from build123d import *

# Parameters (mm, degrees)
F1_DEPTH = 944.626
F2_W     = 12.7
F2_H     = 838.2
F3_DEPTH = 349.25
F4_W     = 368.3
F4_H     = 184.15
F4_R     = 20.6375
F4_W_2   = 247.65
F5_DEPTH = 25.4


with BuildPart() as f1:
    # F0 (on Right) → F1 (new body, symmetric)
    with BuildSketch(Plane.YZ):
        with BuildLine():
            Line((400.05, 361.95), (0, 361.95))
            Line((0, 361.95), (-400.05, 361.95))
            ThreePointArc((-400.05, 361.95), (-422.50064, 352.65064), (-431.8, 330.2))
            Line((-431.8, 330.2), (-431.8, 31.75))
            ThreePointArc((-431.8, 31.75), (-437.379616, 18.279616), (-450.85, 12.7))
            Line((-450.85, 12.7), (-558.8, 12.7))
            Line((-558.8, 12.7), (-558.8, 6.35))
            Line((-558.8, 6.35), (-558.8, 0))
            Line((-558.8, 0), (-450.85, 0))
            ThreePointArc((-450.85, 0), (-428.39936, 9.29936), (-419.1, 31.75))
            Line((-419.1, 31.75), (-419.1, 330.2))
            ThreePointArc((-419.1, 330.2), (-413.520384, 343.670384), (-400.05, 349.25))
            Line((-400.05, 349.25), (0, 349.25))
            Line((0, 349.25), (400.05, 349.25))
            ThreePointArc((400.05, 349.25), (413.520384, 343.670384), (419.1, 330.2))
            Line((419.1, 330.2), (419.1, 31.75))
            ThreePointArc((419.1, 31.75), (428.39936, 9.29936), (450.85, 0))
            Line((450.85, 0), (558.8, 0))
            Line((558.8, 0), (558.8, 6.35))
            Line((558.8, 6.35), (558.8, 12.7))
            Line((558.8, 12.7), (450.85, 12.7))
            ThreePointArc((450.85, 12.7), (437.379616, 18.279616), (431.8, 31.75))
            Line((431.8, 31.75), (431.8, 330.2))
            ThreePointArc((431.8, 330.2), (422.50064, 352.65064), (400.05, 361.95))
        make_face()
    extrude(amount=F1_DEPTH, both=True)

    # F2 (on face) → F3 (join, through all)
    with BuildSketch(Plane(origin=(0, 0, 349.25), x_dir=(1, 0, 0), z_dir=(0, 0, -1))):
        with Locations((757.428, 0)):
            Rectangle(F2_W, F2_H)
    extrude(amount=F3_DEPTH)

    # F4 (on face) → F5 (join)
    with BuildSketch(Plane.XY.offset(361.95)):
        with Locations((-433.324, 301.625)):
            Rectangle(F4_W, F4_H)
        with Locations((-484.124, 317.5)):
            Circle(F4_R, mode=Mode.SUBTRACT)
        with Locations((338.201, 301.625)):
            Rectangle(F4_W_2, F4_H)
        with Locations((328.676, 317.5)):
            Circle(F4_R, mode=Mode.SUBTRACT)
        with Locations((338.201, -301.625)):
            Rectangle(F4_W_2, F4_H)
        with Locations((328.676, -317.5)):
            Circle(F4_R, mode=Mode.SUBTRACT)
        with Locations((-433.324, -301.625)):
            Rectangle(F4_W, F4_H)
        with Locations((-484.124, -317.5)):
            Circle(F4_R, mode=Mode.SUBTRACT)
    extrude(amount=F5_DEPTH)


solid = f1.part
Work out the finished part from the listing and answer in its coordinate system (mm). A direction names the side the tool comes from. Round coordinates to 2 decimals unless told otherwise and drop trailing zeros. Loops run counter-clockwise (first coordinate to the right, second up) from the corner with the lowest first, then second, coordinate; pieces in that order, holes last. Notation, with made-up numbers: (72, -22.5) - (108, -22.5) arc R20 ccw to (108, 14.5) - close; hole circle Ø5 at (50, 39.25). An arc over 180 degrees is marked (long way). One line per item, written item: value.
Q1. Find section A-A on x = -57.5. Give the vertices of the cut face in (y, z).
Check values:
outline: (-558.8, 0) - (-450.85, 0) arc R31.75 ccw to (-419.1, 31.75) - (-419.1, 330.2) arc R19.05 cw to (-400.05, 349.25) - (400.05, 349.25) arc R19.05 cw to (419.1, 330.2) - (419.1, 31.75) arc R31.75 ccw to (450.85, 0) - (558.8, 0) - (558.8, 12.7) - (450.85, 12.7) arc R19.05 cw to (431.8, 31.75) - (431.8, 330.2) arc R31.75 ccw to (400.05, 361.95) - (-400.05, 361.95) arc R31.75 ccw to (-431.8, 330.2) - (-431.8, 31.75) arc R19.05 cw to (-450.85, 12.7) - (-558.8, 12.7) - close
Q2. Each of these flat-tipped pins is pushed along its axis until it touches: pin 1 Ø20.5 at (y, z) = (269.5, 373.5) entering from -X; pin 2 Ø12 at (x, z) = (609.5, 291) entering from +Y; pin 3 Ø20.5 at (y, z) = (345, 372) entering from -X; pin 4 Ø7.5 at (y, z) = (300, 370.5) entering from +X. Where does it stop, or does it pass through?
Check values:
pin 1: x = -617.47
pin 2: y = 431.8
pin 3: x = -944.63
pin 4: x = 462.03
Q3. Straight lines are drawn through the part: probe 1 along X at (y, z) = (317, 369); probe 2 along Y at (x, z) = (-477, 133); probe 3 along Y at (x, z) = (-735, 333). For each, find the intervals that lie inside material, in ascending order.
Check values:
probe 1: -617.47 to -504.76, -463.49 to -249.17, 214.38 to 308.04, 349.31 to 462.03
probe 2: -431.8 to -419.1, 419.1 to 431.8
probe 3: -431.68 to -418.89, 418.89 to 431.68
Q4. For faces 4 (the flat face through (13, -504, 12.7)), 5 (the flat face through (13, 506, 12.7)), 6 (the flat face through (751.078, 6, 177)), determine the directions among +Z, -Z, +X, -X, +Y, -Y from which every point of the face is accessible in a straight line to the end or side of a thin tool.
Check values:
face 4: +Z, +X, -X, -Y
face 5: +Z, +X, -X, +Y
face 6: -Z, -X
Q5. Find section B-B on z = 88.5. Give the vertices of the cut face in (x, y), and give its area (3 significant figures).
Check values:
outline: (-944.63, -431.8) - (944.63, -431.8) - (944.63, -419.1) - (763.78, -419.1) - (763.78, 419.1) - (944.63, 419.1) - (944.63, 431.8) - (-944.63, 431.8) - (-944.63, 419.1) - (751.08, 419.1) - (751.08, -419.1) - (-944.63, -419.1) - close
area: 58,600 mm2
Q6. Find section C-C on y = 317.5. Give the vertices of the cut face in (x, z), and give its area (3 significant figures).
Check values:
outline: (-944.63, 349.25) - (751.08, 349.25) - (751.08, 0) - (763.78, 0) - (763.78, 349.25) - (944.63, 349.25) - (944.63, 361.95) - (462.03, 361.95) - (462.03, 387.35) - (349.31, 387.35) - (349.31, 361.95) - (308.04, 361.95) - (308.04, 387.35) - (214.38, 387.35) - (214.38, 361.95) - (-249.17, 361.95) - (-249.17, 387.35) - (-463.49, 387.35) - (-463.49, 361.95) - (-504.76, 361.95) - (-504.76, 387.35) - (-617.47, 387.35) - (-617.47, 361.95) - (-944.63, 361.95) - close
area: 42,000 mm2
Q7. Find section D-D on y = -57.5. Give the vertices of the cut face in (x, z).
Check values:
outline: (-944.63, 349.25) - (751.08, 349.25) - (751.08, 0) - (763.78, 0) - (763.78, 349.25) - (944.63, 349.25) - (944.63, 361.95) - (-944.63, 361.95) - close
Q8. The mould has two halves that part along X. Classify faces 1 (the flat face through (13, 504, 0)), 2 (the flat face through (944.626, -3, 356)), 3 (the flat face through (-484, 318, 361.95)): +X half, -X half, draft (parallel to the pull), parting line (faces both ways), or undercut.
Check values:
face 1: draft
face 2: +X half
face 3: undercut
